Autodesk Inventor part; units mm, degrees
ref_plane "YZ Plane" through (0, 0, 0) normal (1, 0, 0) x (0, 1, 0)
ref_plane "XZ Plane" through (0, 0, 0) normal (0, 1, 0) x (-1, 0, 0)
ref_plane "XY Plane" through (0, 0, 0) normal (0, 0, 1) x (1, 0, 0)
sketch "Sketch1" plane through (0, 0, 0) normal (0, 1, 0) x (-1, 0, 0)
  line L0 (-14, 34.5) -> (12.387, 34.5)
  line L1 (12.387, 34.5) -> (12.387, -30.5)
  line L2 (12.387, -30.5) -> (-14, -30.5)
  line L3 (-14, -30.5) -> (-14, 34.5)
  dimension "d0" = 26.387
  dimension "d1" = 65
extrude "Extrusion1" add sketch "Sketch1" along normal blind 5
fillet "Fillet1" radius 5 2 edges at (14, 2.5, 34.5) (14, 2.5, -30.5)
sketch "Sketch2" plane through (0, 5, 0) normal (0, 1, 0) x (1, 0, 0)
  line L0 (-9, -34.5716) -> (-9, -26.4716)
  line L1 (-9, -26.4716) -> (-0.5, -26.4716)
  line L2 (-0.5, -26.4716) -> (-0.5, -34.5716)
  line L3 (-0.5, -34.5716) -> (-9, -34.5716)
  point P0 (0, 0)
  point P1 (-12.387, -34.5)
  dimension "d6" = 8.1
  dimension "d7" = 8.5
extrude "Extrusion2" cut sketch "Sketch2" against normal through all
sketch "Sketch3" plane through (0, 5, 0) normal (0, 1, 0) x (1, 0, 0)
  line L0 (14, -27.8288) -> (3, -27.8288)
  line L1 (3, -27.8288) -> (3, -10.8288)
  line L2 (3, -10.8288) -> (14, -10.8288)
  line L3 (14, -10.8288) -> (14, -27.8288)
  line L4 (14, 6.0005) -> (3, 6.0005)
  line L5 (3, 6.0005) -> (3, 23.0005)
  line L6 (3, 23.0005) -> (14, 23.0005)
  line L7 (14, 23.0005) -> (14, 6.0005)
  point P0 (0, 0)
  dimension "d12" = 11
  dimension "d13" = 17
  dimension "d22" = 11
  dimension "d23" = 17
extrude "Extrusion3" cut sketch "Sketch3" against normal through all
sketch "Sketch4" plane through (0, 5, 0) normal (0, 1, 0) x (1, 0, 0)
  line L0 (14, 6.0005) -> (3, 6.0005)
  line L1 (3, 23.0005) -> (3, 6.0005)
  line L2 (2.1408, 15.4204) -> (-5.4822, 15.4204)
  line L3 (-5.4822, 15.4204) -> (-5.4822, 1.2634)
  line L4 (-5.4822, 1.2634) -> (2.1408, 1.2634)
  line L5 (2.1408, 1.2634) -> (2.1408, 15.4204)
  line L6 (-12.387, 30.5) -> (-12.387, -34.5)
  line L7 (-10.912, 29.3102) -> (-2, 29.3102)
  line L8 (-2, 29.3102) -> (-2, 20.3982)
  line L9 (-2, 20.3982) -> (-10.912, 20.3982)
  line L10 (-10.912, 20.3982) -> (-10.912, 29.3102)
  point P0 (0, 0)
  dimension "d29" = 7.623
  dimension "d30" = 14.157
  dimension "d33" = 8.912
  dimension "d34" = 8.912
extrude "Extrusion4" cut sketch "Sketch4" against normal through all
properties part number "Charger_support"
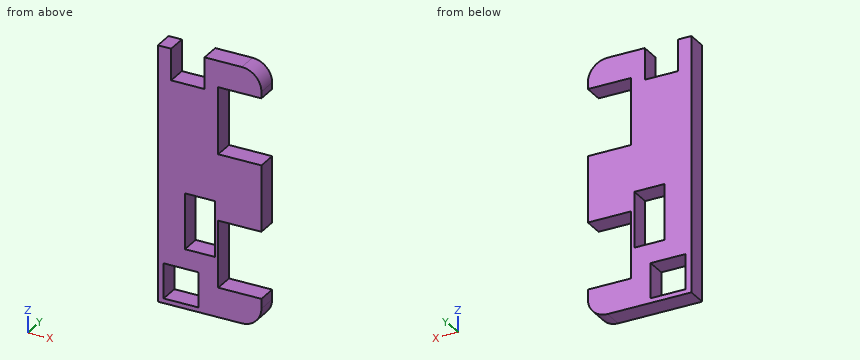
CAD build for the part. Positions are in the model's coordinates, mm. Coordinates: 2 decimals unless noted, no trailing zeros. Write each loop counter-clockwise with the first axis right and the second up, starting at its lowest first coordinate (ties: lowest second). Pieces come first, ordered by that corner, then holes. Notation, with made-up numbers: (62, 68) -> (102, 68) arc R28 ccw to (102, 104) -> close; hole circle Ø5 at (36.5, 85). An arc over 180 degrees is marked (long way). Return JSON: item names as keys, results as strings. Group by question number.
Q1. Drill centre lines: line 1 (Z direction, x = -4.5, y = 1.8); line 2 (Z direction, x = 4.25, y = 3.65); line 3 (X direction, y = 1.85, z = -25.5). Where is each one in solid material? Low to high.
Q2. Cut at C-C, the plane y = 2.2. Give the cut face in (x, z), then the cut area to 3 significant figures.
Q3. Flat gauge pins, fed straight in: pin 1 (2 mm diameter, centred on x = -2.5, y = 0.5, fed in from +Z); pin 2 (1.5 mm diameter, centred on y = 0.5, z = 19, fed in from +X). Where does each tip first touch, or does it go through?
Q4. Cut at D-D, the plane x = 5.5. Give the cut face in (y, z), then the cut area to 3 significant figures.
Q5. Cut at B-B, the plane z = -12. Give the cut face in (x, y).
Q6. Cut at A-A, the plane x = -6.5. Give the cut face in (y, z), then the cut area to 3 significant figures.
Returned:
{
 "1": {"line 1": "z = -30.5 to -29.31, -20.4 to -15.42, -1.26 to 26.47", "line 2": "z = -30.5 to -23, -6 to 10.83, 27.83 to 34.5", "line 3": "x = -12.39 to -10.91, -2 to 14"},
 "2": {"outline": "(-12.39, -30.5) -> (9, -30.5) arc R5 ccw to (14, -25.5) -> (14, -23) -> (3, -23) -> (3, -6) -> (14, -6) -> (14, 10.83) -> (3, 10.83) -> (3, 27.83) -> (14, 27.83) -> (14, 29.5) arc R5 ccw to (9, 34.5) -> (-0.5, 34.5) -> (-0.5, 26.47) -> (-9, 26.47) -> (-9, 34.5) -> (-12.39, 34.5) -> close; hole (-10.91, -29.31) -> (-2, -29.31) -> (-2, -20.4) -> (-10.91, -20.4) -> close; hole (-5.48, -15.42) -> (2.14, -15.42) -> (2.14, -1.26) -> (-5.48, -1.26) -> close", "area": "1,070 mm2"},
 "3": {"pin 1": "stops at z = 26.47", "pin 2": "stops at x = 3"},
 "4": {"outline": "(0, -30.5) -> (5, -30.5) -> (5, -23) -> (0, -23) -> close; (0, -6) -> (5, -6) -> (5, 10.83) -> (0, 10.83) -> close; (0, 27.83) -> (5, 27.83) -> (5, 34.5) -> (0, 34.5) -> close", "area": "155 mm2"},
 "5": {"outline": "(-12.39, 0) -> (-5.48, 0) -> (-5.48, 5) -> (-12.39, 5) -> close; (2.14, 0) -> (3, 0) -> (3, 5) -> (2.14, 5) -> close"},
 "6": {"outline": "(0, -30.5) -> (5, -30.5) -> (5, -29.31) -> (0, -29.31) -> close; (0, -20.4) -> (5, -20.4) -> (5, 26.47) -> (0, 26.47) -> close", "area": "240 mm2"}
}
